Study the drawing (mm; zero at the part's minimum x, y, z) and answer. A direction names the side the tool comes from. Round coordinates to 2 decimals unless told otherwise and drop trailing zeros. Write each loop counter-clockwise with the first axis right and the second up, starting at its lowest first coordinate (ties: lowest second). Pieces come first, ordered by that corner, then holes. Notation, with made-up numbers: M 54,49.25 L 70,49.25 A26 cw 70,74.25 Z; hole C 39,-26 d9. An arc over 180 degrees is marked long. Write each question's results on one line, items separated by ' | '.
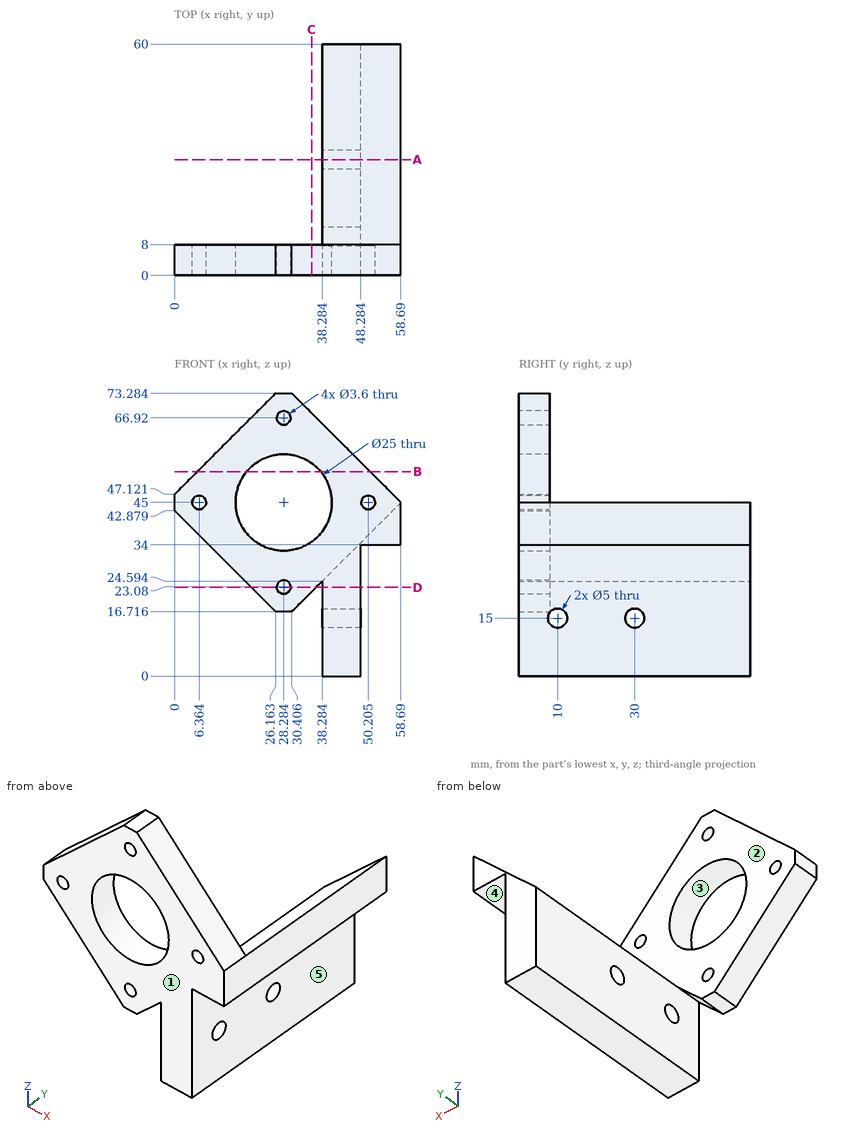
1) Section D-D (z = 23) is taken. Determine the outline of the cut face in (x, y) (1 decimal), then the cut area to 3 significant figures.
Return value:
outline: M 19.9,0 L 26.5,0 L 26.5,8 L 19.9,8 Z; M 30.1,0 L 36.7,0 L 36.7,8 L 30.1,8 Z; M 38.3,0 L 48.3,0 L 48.3,60 L 38.3,60 Z | area: 706 mm²
2) A tool of negligible diameter and unlimited length cuts with its end or side. For the marked faces 1 and 2, from which of +Z, -Z, +X, -X, +Y, -Y can it reach the whole face along a straight path? Write none if from no direction.
Return value:
face 1: +Z, -Z, +X, -X, -Y | face 2: +Z, -X, +Y
3) Each of these flat-tipped pins is pushed along its axis until it touches: pin 1 (4.5 mm diameter, centred on x = 50.2, z = 45, fed in from +Y); pin 2 (2 mm diameter, centred on x = 29.5, y = 2.5, fed in from -Z); pin 3 (12.5 mm diameter, centred on y = 24, z = 9, fed in from -X). Where does it stop, or does it pass through?
Return value:
pin 1: y = 8 | pin 2: z = 16.72 | pin 3: x = 38.28
4) Section B-B (z = 53) is taken. Determine the outline of the cut face in (x, y).
Return value:
outline: M 5.88,0 L 18.68,0 L 18.68,8 L 5.88,8 Z; M 37.89,0 L 50.69,0 L 50.69,8 L 37.89,8 Z
5) Section A-A (y = 30) is taken. Determine the outline of the cut face in (x, z) (1 decimal), then the cut area to 3 significant figures.
Return value:
outline: M 38.3,0 L 48.3,0 L 48.3,12.5 L 38.3,12.5 Z; M 38.3,17.5 L 48.3,17.5 L 48.3,34 L 58.7,34 L 58.7,45 L 38.3,24.6 Z | area: 306 mm²
6) The mould has two halves that part along Z. Classify the marked faces 3, 4 and 5: +Z half, -Z half, draft (parallel to the pull), parting line (faces both ways), or undercut.
Return value:
face 3: undercut | face 4: -Z half | face 5: draft
7) Find the intervals of material crossed by line 1 (Y direction, x = 43, z = 15); line 2 (X direction, y = 2.5, z = 45) (1 decimal); line 3 (Y direction, x = 9, z = 49.5), in increasing order.
Return value:
line 1: 0 to 7.5, 12.5 to 27.5, 32.5 to 60 | line 2: 0 to 4.6, 8.2 to 15.8, 40.8 to 48.4, 52 to 58.7 | line 3: 0 to 8
8) Section C-C (x = 35.5) is taken. Determine the outline of the cut face in (y, z).
Return value:
outline: M 0,21.81 L 8,21.81 L 8,34.79 L 0,34.79 Z; M 0,55.21 L 8,55.21 L 8,68.19 L 0,68.19 Z
